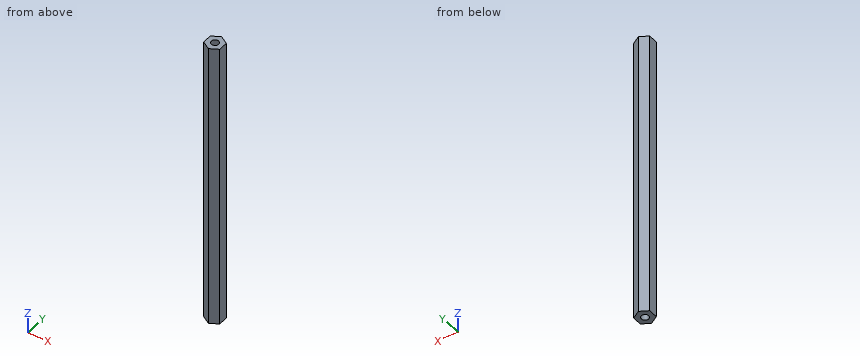
Autodesk Inventor part; units mm, degrees
ref_plane "YZ Plane" through (0, 0, 0) normal (1, 0, 0) x (0, 1, 0)
ref_plane "XZ Plane" through (0, 0, 0) normal (0, 1, 0) x (-1, 0, 0)
ref_plane "XY Plane" through (0, 0, 0) normal (0, 0, 1) x (1, 0, 0)
sketch "スケッチ1" plane through (0, 0, 0) normal (0, 0, 1) x (1, 0, 0)
  line L0 (0, 3.1754) -> (2.75, 1.5877)
  line L1 (2.75, 1.5877) -> (2.75, -1.5877)
  line L2 (2.75, -1.5877) -> (0, -3.1754)
  line L3 (0, -3.1754) -> (-2.75, -1.5877)
  line L4 (-2.75, -1.5877) -> (-2.75, 1.5877)
  line L5 (-2.75, 1.5877) -> (0, 3.1754)
  point P0 (0, 0)
  point P1 (0, 0)
  dimension "d0" = 5.5
extrude "押し出し1" add sketch "スケッチ1" along normal blind 100
sketch "スケッチ2" plane through (0, 0, 100) normal (0, 0, 1) x (1, 0, 0)
  point P0 (0, 0)
hole "穴1" at (0, 0, 100) direction (0, 0, -1) diameter 2.459 depth 8.8 tip angle 118
sketch "スケッチ3" plane through (0, 0, 0) normal (0, 0, -1) x (-1, 0, 0)
  point P0 (0, 0)
hole "穴2" at (0, 0, 0) direction (0, 0, 1) diameter 2.459 depth 8.8 tip angle 118
properties part number "アルミスペーサー(六角・酸洗処理）_ASL-3100E" material "アルミニウム 6061"
Geometry check sheet. Reference: the model listing, model coordinates, mm. Coordinates: 2 decimals unless noted, no trailing zeros. Order: outer loops, then holes, each group sorted by start corner. A loop starts at its lowest first (then second) coordinate and runs counter-clockwise, first axis right, second up. Notation, with made-up numbers: M 84,6.5 L 90,6.5 A37 cw 90,42.5 Z; hole C 74.5,-27 d11. An arc over 180 degrees is marked long. Use CSV: the item, a comma, the result in double quotes.
Item 1: Cross-section at A-A on z = 74. Record the cut outline in (x, y).
Returned:
outline,"M -2.75,-1.59 L 0,-3.18 L 2.75,-1.59 L 2.75,1.59 L 0,3.18 L -2.75,1.59 Z"
Item 2: Gauge pin test, flat ends, axial feed: pin 1 Ø1 at (x, z) = (-1, 66) entering from -Y; pin 2 Ø1.5 at (x, y) = (0, 0) entering from -Z. Record the tip position at first contact, or that the pin passes through.
Returned:
pin 1,"stops at y = -2.89"
pin 2,"stops at z = 9.09"
Item 3: Thickness scan on line 1 along X through (y, z) = (0, 3.5); line 2 along Y through (x, z) = (0, 95.75); line 3 along X through (y, z) = (0.5, 7.5). Record the ranges inside material, lowest first.
Returned:
line 1,"x = -2.75 to -1.23, 1.23 to 2.75"
line 2,"y = -3.18 to -1.23, 1.23 to 3.18"
line 3,"x = -2.75 to -1.12, 1.12 to 2.75"
